Could you check a few things on this drawing? It's one solid part, dimensions in mm from its lowest x, y, z. A direction names the side the tool comes from. Give positions to 0.01 mm unless a question says otherwise; leave off trailing zeros. Order: outer loops, then holes, each group sorted by start corner. A loop starts at its lowest first (then second) coordinate and runs counter-clockwise, first axis right, second up. Notation, with made-up numbers: M 86.5,-35.5 L 124.5,-35.5 A24 ccw 124.5,-21.5 Z; hole C -39,83 d9. An arc over 180 degrees is marked long. Use CSV: the item, a comma, the result in double quotes. Start each with the question number.
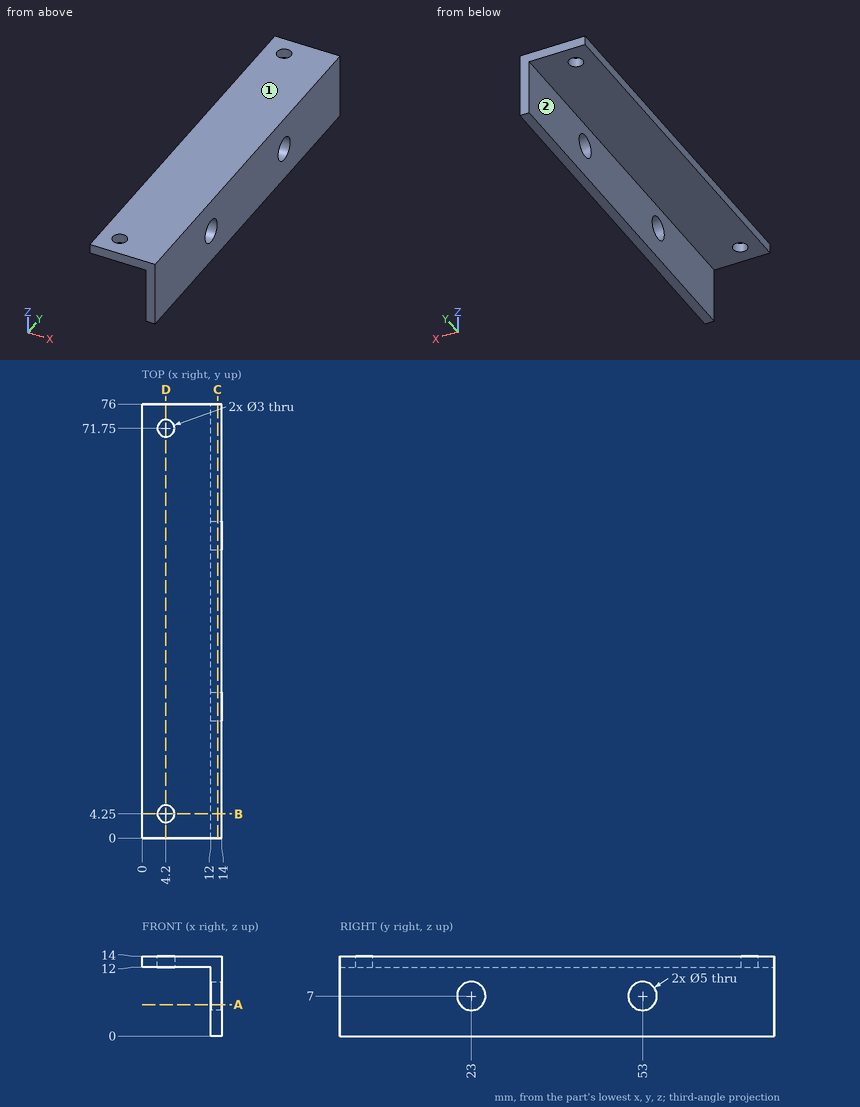
Q1. For the marked faces 1 and 2, which set-ups out of +Z, -Z, +X, -X, +Y, -Y let a thin tool reach every point of the face, with its end or its side?
Q2. Imagine slicing it at B-B, the plane y = 4.25. Please give me the cut outline in (x, z).
Q3. Imagine slicing it at A-A, the plane z = 5.5. Please give me the cut outline in (x, y), then the cut area to 3 significant figures.
Q4. I need wall thicknesses on line 1 (Y direction, x = 13.3, z = 7); line 2 (Y direction, x = 4.2, z = 13); line 3 (X direction, y = 71.75, z = 13.1). Which ranges of each line are inside material? Lowest first, please. Write a range as [from, to].
Q5. Imagine slicing it at D-D, the plane x = 4.2. Please give me the cut outline in (y, z), then the cut area to 3 significant figures.
Q6. For P1, Ø3, axis at y = 49.5, z = 2, coming from the -X side; P2, Ø1.5, axis at x = 3, y = 60, coming from the -Z side, each with a flat end and sliding along its axis, tell me the tip position at first contact or that it passes through.
Q7. Imagine slicing it at C-C, the plane x = 13.25. Please give me the cut outline in (y, z).
Reply:
1,face 1,"+Z, +X, -X, +Y, -Y"
1,face 2,"-Z, -X, +Y, -Y"
2,outline,"M 0,12 L 2.7,12 L 2.7,14 L 0,14 Z; M 5.7,12 L 12,12 L 12,0 L 14,0 L 14,14 L 5.7,14 Z"
3,outline,"M 12,0 L 14,0 L 14,21 L 12,21 Z; M 12,25 L 14,25 L 14,51 L 12,51 Z; M 12,55 L 14,55 L 14,76 L 12,76 Z"
3,area,"136 mm^2"
4,line 1,"y = [0, 20.5], [25.5, 50.5], [55.5, 76]"
4,line 2,"y = [0, 2.75], [5.75, 70.25], [73.25, 76]"
4,line 3,"x = [0, 2.7], [5.7, 14]"
5,outline,"M 0,12 L 2.75,12 L 2.75,14 L 0,14 Z; M 5.75,12 L 70.25,12 L 70.25,14 L 5.75,14 Z; M 73.25,12 L 76,12 L 76,14 L 73.25,14 Z"
5,area,"140 mm^2"
6,P1,"stops at x = 12"
6,P2,"stops at z = 12"
7,outline,"M 0,0 L 76,0 L 76,14 L 0,14 Z; hole C 23,7 d5; hole C 53,7 d5"
